Source: CAD feature listing. Evaluate the final solid. Frame: model axes, mm. Face numbers are marked on the shaded views. Coordinates: 2 decimals unless noted, no trailing zeros. Order: outer loops, then holes, each group sorted by start corner. A loop starts at its lowest first (then second) coordinate and runs counter-clockwise, first axis right, second up.
Item 1: Contact query for flat-ended pins moving along their axis: P1, Ø6, axis at y = -27.5, z = 64.5, coming from the -X side; P2, Ø6, axis at y = 28, z = 47, coming from the +X side; P3, Ø1.5, axis at x = -24.5, y = 5.5, coming from the -Z side; P4, Ø2.5, axis at x = 75.5, z = 12.5, coming from the +Y side. Output: stop coordinate, or through.
Item 2: Section A-A on x = 0. Return the cut outline in (y, z).
Item 3: Section B-B on y = 11.5. Return the cut outline in (x, z), then the cut area to 3 significant figures.
Item 4: Ray query, line 1 (Z direction, x = 52, y = -59); line 2 (X direction, y = 17.5, z = 6); line 3 (Y direction, x = 67, z = 42.5). Return the intervals inside material, ascending.
Item 5: Section C-C on z = 56. Return the cut outline in (x, y).
Item 6: Mould query, pull axis Y, two halves, no side actions, for the marked faces 1, 2, 3 and 4. Classes: released by +Y, released by -Y, zero draft, split by the parting line, or undercut.
Item 7: Section D-D on x = -16.5. Return the cut outline in (y, z), then the cut area to 3 significant figures.
from build123d import *

# Parameters (mm, degrees)
F0_W     = 150.186099
F0_H     = 95.117865
F1_DEPTH = 20
F2_R     = 7.844958
F3_DEPTH = 70
F4_W     = 149.729192
F4_H     = 20.198451
F5_DEPTH = 100


with BuildPart() as f1:
    # F0 (on Top) → F1 (new body)
    with BuildSketch(Plane.XY):
        with Locations((1.266945, -27.573706)):
            Rectangle(F0_W, F0_H)
    extrude(amount=F1_DEPTH)

    # F2 (on face) → F3 (join)
    with BuildSketch(Plane.XY.offset(20)):
        with Locations((0, -36.366057)):
            Circle(F2_R)
    extrude(amount=F3_DEPTH)

    # F4 (on Top) → F5 (join)
    with BuildSketch(Plane.XY):
        with Locations((-0.657424, 28.801786)):
            Rectangle(F4_W, F4_H)
    extrude(amount=F5_DEPTH)


solid = f1.part
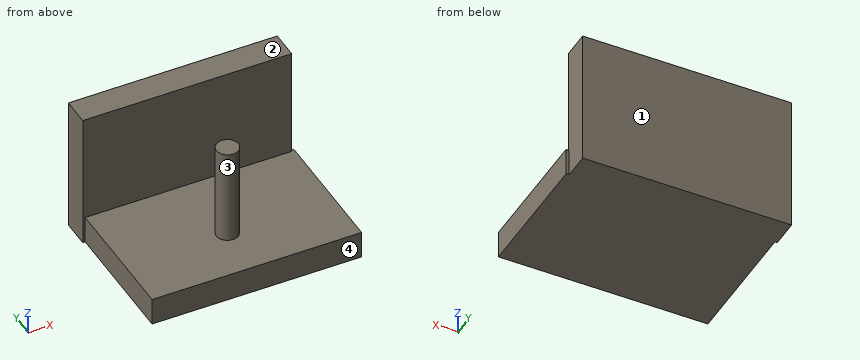
Answer list:
1. P1: stops at x = -5.21
1. P2: stops at x = 74.21
1. P3: stops at z = 0
1. P4: stops at y = 19.99
2. outline: (-75.13, 0) - (38.9, 0) - (38.9, 100) - (18.7, 100) - (18.7, 20) - (-28.52, 20) - (-28.52, 90) - (-44.21, 90) - (-44.21, 20) - (-75.13, 20) - close
3. outline: (-73.83, 0) - (76.36, 0) - (76.36, 20) - (-73.83, 20) - close
3. area: 3,000 mm2
4. line 1: z = 0 to 20
4. line 2: x = -73.83 to 76.36
4. line 3: y = 18.7 to 38.9
5. outline: (-75.52, 18.7) - (74.21, 18.7) - (74.21, 38.9) - (-75.52, 38.9) - close; circle Ø15.69 at (0, -36.37)
6. face 1: released by +Y
6. face 2: zero draft
6. face 3: undercut
6. face 4: released by -Y
7. outline: (-75.13, 0) - (38.9, 0) - (38.9, 100) - (18.7, 100) - (18.7, 20) - (-75.13, 20) - close
7. area: 3,900 mm2
